Autodesk Inventor part; units mm, degrees
ref_plane "YZ Plane" through (0, 0, 0) normal (1, 0, 0) x (0, 1, 0)
ref_plane "XZ Plane" through (0, 0, 0) normal (0, 1, 0) x (-1, 0, 0)
ref_plane "XY Plane" through (0, 0, 0) normal (0, 0, 1) x (1, 0, 0)
sketch "草图1" plane through (0, 0, 0) normal (0, 0, 1) x (1, 0, 0)
  line L0 (-144.4444, 0) -> (-144.4444, 58)
  line L1 (-144.4444, 58) -> (-122.4444, 58)
  line L2 (-122.4444, 58) -> (-122.4444, 32)
  line L3 (-122.4444, 32) -> (-41.9444, 32)
  line L4 (-41.9444, 32) -> (-41.9444, 65)
  line L5 (-41.9444, 65) -> (-4.9444, 65)
  line L6 (-4.9444, 65) -> (-4.9444, 38)
  line L7 (-4.9444, 38) -> (30.0556, 38)
  line L8 (30.0556, 38) -> (30.0556, 0)
  line L9 (0, 0) -> (-166.6667, 0) construction
  line L10 (-144.4444, 0) -> (-144.4444, -58)
  line L11 (-144.4444, -58) -> (-122.4444, -58)
  line L12 (-122.4444, -58) -> (-122.4444, -32)
  line L13 (-122.4444, -32) -> (-41.9444, -32)
  line L14 (-41.9444, -32) -> (-41.9444, -65)
  line L15 (-41.9444, -65) -> (-4.9444, -65)
  line L16 (-4.9444, -65) -> (-4.9444, -38)
  line L17 (-4.9444, -38) -> (30.0556, -38)
  line L18 (30.0556, -38) -> (30.0556, 0)
  circle A0 centre (-106.5528, 0) radius 7.5
  circle A1 centre (-64.5976, 0) radius 7.5
  point P0 (-141.4444, -54)
  point P1 (-127.4444, -54)
  point P2 (-27.9137, -54)
  point P3 (-14.1378, -54)
  point P4 (-112.1204, -28)
  point P5 (-64.5976, -28)
  point P6 (-89.6514, -28)
  point P7 (-127.4444, -38)
  point P8 (-141.4444, -38)
  point P9 (-27.9137, -38)
  point P10 (-14.3619, -38)
  point P11 (-141.4444, 54)
  point P12 (-127.4444, 54)
  point P13 (-127.4444, 38)
  point P14 (-141.4444, 38)
  point P15 (-27.9137, 54)
  point P16 (-27.9137, 38)
  point P17 (-14.1378, 54)
  point P18 (-14.3619, 38)
  point P19 (-64.5976, 28)
  point P20 (-89.6514, 28)
  point P21 (-112.1204, 28)
  point P22 (-133.4444, 58)
  point P23 (-23.4444, 65)
  dimension "d0" = 22
  dimension "d1" = 37
  dimension "d3" = 32
  dimension "d4" = 38
  dimension "d5" = 35
  dimension "d6" = 58
  dimension "d7" = 15
  dimension "d8" = 15
  dimension "d29" = 28
  dimension "d30" = 28
  dimension "d31" = 28
  dimension "d36" = 110
  dimension "d96" = 33
extrude "拉伸1" add sketch "草图1" along normal blind 5
sketch "草图2" plane through (0, 0, 5) normal (0, 0, 1) x (1, 0, 0)
  circle A0 centre (-64.5976, 0) radius 7.5 construction
  circle A1 centre (-106.5528, 0) radius 7.5 construction
  line L0 (-144.4444, -58) -> (-144.4444, 58) construction
  line L1 (-144.4444, 58) -> (-122.4444, 58) construction
  line L2 (-122.4444, 58) -> (-122.4444, 32) construction
  line L3 (-122.4444, 32) -> (-41.9444, 32) construction
  line L4 (-41.9444, 32) -> (-41.9444, 65) construction
  line L5 (-41.9444, 65) -> (-4.9444, 65) construction
  line L6 (-4.9444, 65) -> (-4.9444, 38) construction
  line L7 (-4.9444, 38) -> (30.0556, 38) construction
  line L8 (30.0556, 38) -> (30.0556, -38) construction
  line L9 (30.0556, -38) -> (-4.9444, -38) construction
  line L10 (-4.9444, -38) -> (-4.9444, -65) construction
  line L11 (-4.9444, -65) -> (-41.9444, -65) construction
  line L12 (-41.9444, -65) -> (-41.9444, -32) construction
  line L13 (-41.9444, -32) -> (-122.4444, -32) construction
  line L14 (-122.4444, -32) -> (-122.4444, -58) construction
  line L15 (-122.4444, -58) -> (-144.4444, -58) construction
  line L16 (-164.7255, 0) -> (-80.9793, 0) construction
  point P0 (0, 0)
  point P1 (-141.4444, 55)
  point P2 (-125.4444, 55)
  point P3 (-38.4444, 61.5)
  point P4 (-8.4444, 61.5)
  point P5 (-38.4444, 37.5)
  point P6 (-8.4444, 37.5)
  point P7 (-125.4444, 41)
  point P8 (-141.4444, 41)
  point P9 (-141.4444, -55)
  point P10 (-125.4444, -55)
  point P11 (-38.4444, -61.5)
  point P12 (-8.4444, -61.5)
  point P13 (-38.4444, -37.5)
  point P14 (-8.4444, -37.5)
  point P15 (-125.4444, -41)
  point P16 (-141.4444, -41)
  dimension "d32" = 3
  dimension "d33" = 3
  dimension "d34" = 16
  dimension "d37" = 3
  dimension "d38" = 14
  dimension "d39" = 3
  dimension "d40" = 14
  dimension "d42" = 30
  dimension "d43" = 30
  dimension "d44" = 24
  dimension "d45" = 3.5
  dimension "d46" = 3.5
  dimension "d47" = 3.5
  dimension "d95" = 16
hole "孔2" at (-141.4444, 55, 5) at (-125.4444, 55, 5) at (-125.4444, 41, 5) at (-141.4444, 41, 5) at (-141.4444, -41, 5) at (-125.4444, -41, 5) at (-125.4444, -55, 5) at (-141.4444, -55, 5) direction (0, 0, -1) diameter 3.6 end through all
sketch "草图3" plane through (0, 0, 5) normal (0, 0, 1) x (1, 0, 0)
  circle A0 centre (-125.4444, -55) radius 1.8 construction
  circle A1 centre (-141.4444, -55) radius 1.8 construction
  circle A2 centre (-125.4444, 41) radius 1.8 construction
  circle A3 centre (-141.4444, 55) radius 1.8 construction
  circle A4 centre (-125.4444, 55) radius 1.8 construction
  circle A5 centre (-141.4444, 41) radius 1.8 construction
  circle A6 centre (-141.4444, -41) radius 1.8 construction
  circle A7 centre (-125.4444, -41) radius 1.8 construction
  circle A8 centre (-64.5976, 0) radius 7.5 construction
  circle A9 centre (-106.5528, 0) radius 7.5 construction
  line L0 (-144.4444, 58) -> (-144.4444, -58) construction
  line L1 (-144.4444, -58) -> (-122.4444, -58) construction
  line L2 (-122.4444, -58) -> (-122.4444, -32) construction
  line L3 (-122.4444, -32) -> (-41.9444, -32) construction
  line L4 (-41.9444, -32) -> (-41.9444, -65) construction
  line L5 (-41.9444, -65) -> (-4.9444, -65) construction
  line L6 (-4.9444, -65) -> (-4.9444, -38) construction
  line L7 (-4.9444, -38) -> (30.0556, -38) construction
  line L8 (30.0556, -38) -> (30.0556, 38) construction
  line L9 (30.0556, 38) -> (-4.9444, 38) construction
  line L10 (-4.9444, 38) -> (-4.9444, 65) construction
  line L11 (-4.9444, 65) -> (-41.9444, 65) construction
  line L12 (-41.9444, 65) -> (-41.9444, 32) construction
  line L13 (-41.9444, 32) -> (-122.4444, 32) construction
  line L14 (-122.4444, 32) -> (-122.4444, 58) construction
  line L15 (-122.4444, 58) -> (-144.4444, 58) construction
  line L16 (0, 0) -> (-184.5407, 0) construction
  point P0 (-139.9444, 25.8646)
  point P1 (-139.9444, 10.9473)
  point P2 (-108.7515, 25.8646)
  point P3 (-89.9847, 25.8646)
  point P4 (-70.7366, 25.8646)
  point P5 (-139.9444, -25.8646)
  point P6 (-139.9444, -10.9473)
  point P7 (-108.7515, -25.8646)
  point P8 (-89.9847, -25.8646)
  point P9 (-70.7366, -25.8646)
  point P10 (-139.9444, 0)
hole "孔3" at (-139.9444, 25.8646, 5) at (-139.9444, -25.8646, 5) at (-139.9444, 0, 5) direction (0, 0, -1) diameter 3.2 end through all
sketch "草图4" plane through (0, 0, 5) normal (0, 0, 1) x (1, 0, 0)
  circle A0 centre (-13.8026, 0) radius 7.5
  line L0 (0, 0) -> (-54.2498, 0) construction
  line L1 (-144.4444, 58) -> (-144.4444, -58) construction
  line L2 (30.0556, -38) -> (30.0556, 38) construction
  point P0 (-19.9444, 18.5)
  point P1 (17.0556, 18.5)
  point P2 (9.0556, 35)
  point P3 (-19.9444, -18.5)
  point P4 (17.0556, -18.5)
  point P5 (9.0556, -35)
  point P6 (-65.2677, 13.1999)
  point P7 (-65.2677, -14.7401)
  dimension "d62" = 15
  dimension "d67" = 37
  dimension "d68" = 50
  dimension "d69" = 18.5
  dimension "d70" = 35
  dimension "d71" = 21
  dimension "d94" = 27.94
extrude "拉伸2" cut sketch "草图4" against normal through all
sketch "草图5" plane through (0, 0, 5) normal (0, 0, 1) x (1, 0, 0)
  line L0 (30.0556, -38) -> (30.0556, 38)
  line L1 (0, 0) -> (-47.6944, 0) construction
  point P0 (26.0556, 29)
  point P1 (-43.9444, 29)
  point P2 (-43.7151, 20)
  point P3 (26.0556, -29)
  point P4 (-43.9444, -29)
  point P5 (-43.7151, -20)
  dimension "d81" = 70
  dimension "d83" = 4
  dimension "d84" = 29
  dimension "d85" = 20
  dimension "d86" = 29
hole "孔5" at (-43.9444, 29, 5) at (-43.9444, -29, 5) at (26.0556, 29, 5) at (26.0556, -29, 5) direction (0, 0, -1) diameter 3.2 end through all
hole "孔6" at (-38.4444, 61.5, 5) at (-8.4444, 61.5, 5) at (-38.4444, 37.5, 5) at (-8.4444, 37.5, 5) at (-38.4444, -37.5, 5) at (-8.4444, -37.5, 5) at (-8.4444, -61.5, 5) at (-38.4444, -61.5, 5) direction (0, 0, -1) diameter 4.2 end through all
sketch "草图6" plane through (0, 0, 5) normal (0, 0, 1) x (1, 0, 0)
  line L0 (-144.4444, 58) -> (-144.4444, -58)
  line L1 (0, 0) -> (-40.7503, 0) construction
  point P0 (-129.4444, 18.5)
  point P1 (-92.4444, 18.5)
  point P2 (-129.4444, -18.5)
  point P3 (-92.4444, -18.5)
  dimension "d104" = 15
  dimension "d105" = 37
  dimension "d106" = 18.5
  dimension "d107" = 18.5
hole "孔7" at (-129.4444, 18.5, 5) at (-92.4444, 18.5, 5) at (-129.4444, -18.5, 5) at (-92.4444, -18.5, 5) direction (0, 0, -1) diameter 3.2 end through all
sketch "草图7" plane through (0, 0, 5) normal (0, 0, 1) x (1, 0, 0)
  point P0 (0, 0)
  point P1 (11.1767, 22.7515)
  point P2 (17.9767, -25.8485)
  point P3 (-62.1233, 22.7515)
  point P4 (-64.6233, -25.2485)
  dimension "d115" = 48.6
  dimension "d116" = 6.8
  dimension "d117" = 73.3
  dimension "d118" = 48
  dimension "d119" = 2.5
hole "孔8" at (-64.6233, -25.2485, 5) at (17.9767, -25.8485, 5) direction (0, 0, -1) diameter 3.2 end through all
sketch "草图8" plane through (0, 0, 5) normal (0, 0, 1) x (1, 0, 0)
  line L0 (30.0556, 38) -> (-4.9444, 38)
  line L1 (0, 0) -> (93.7016, 0) construction
  line L2 (30.0556, -38) -> (30.0556, 38)
  line L3 (-41.9444, 32) -> (-122.4444, 32)
  point P0 (5.0556, 29)
  point P1 (-9.9444, 29)
  point P2 (5.0556, -29)
  point P3 (-9.9444, -29)
  point P4 (-111.5097, 25)
  point P5 (-111.5097, -25)
  dimension "d127" = 15
  dimension "d128" = 9
  dimension "d129" = 9
  dimension "d137" = 25
  dimension "d138" = 7
hole "孔9" at (5.0556, 29, 5) at (-9.9444, 29, 5) at (-9.9444, -29, 5) at (5.0556, -29, 5) at (-111.5097, 25, 5) at (-111.5097, -25, 5) direction (0, 0, -1) diameter 3.2 end through all
properties part number "底盘4.0" material "尼龙 6/6"
Could you check a few things on this model? Use its own coordinates, in mm. A direction names the side the tool comes from. Give positions to 0.01 mm unless a question says otherwise; leave off trailing zeros. Loops run counter-clockwise (first coordinate to the right, second up) from the corner with the lowest first, then second, coordinate; pieces in that order, holes last. Notation, with made-up numbers: (-7.75, 37.5) -> (9.25, 37.5) arc R18 cw to (9.25, 43.5) -> close; hole circle Ø6 at (-4.75, 41). An arc over 180 degrees is marked (long way). Return JSON: item names as keys, results as strings.
Item 1: If we section it at C-C on z = 2.45: Count the separate pieces of the cut face and the enclosed holes in it, plus the area to 3 significant figures.
Geometry results:
{"separate pieces": "1", "enclosed holes": "38", "area": "14,300 mm²"}
Item 2: Which directions (+Z, -Z, +X, -X, +Y, -Y) give clear straight access to the entire face, cutting with the end or side of a thin tool? Please do faces 1 (the flat face through (-41.944, -48, 2)), 2 (the cylindrical face through (-139.687, 55.39, 2.465)), 3 (the flat face through (-134, 58, 2)).
Geometry results:
{"face 1": "+Z, -Z, -Y", "face 2": "+Z, -Z", "face 3": "+Z, -Z, -X, +Y"}
Item 3: I'm going to push flat-ended pins straight in: pin 1 (2.5 mm diameter, centred on x = -91.5, z = 2, fed in from -Y); pin 2 (1.9 mm diameter, centred on x = 26.06, y = -29, fed in from +Z); pin 3 (1.5 mm diameter, centred on x = 9.5, z = 1.5, fed in from +Y). Where does each tip first touch, or does it pass through?
Geometry results:
{"pin 1": "stops at y = -32", "pin 2": "passes through", "pin 3": "stops at y = 38"}
Item 4: I need wall thicknesses on L1, parallel to X at y = 55, z = 2.75; L2, parallel to X at y = 37.5, z = 4.2; L3, parallel to Y at x = -38.5, z = 2.1. Which ranges of each line are inside material? Lowest first, please. Write a range as from..to.
Geometry results:
{"L1": "x = -144.44..-143.24, -139.64..-127.24, -123.64..-122.44, -41.94..-4.94", "L2": "x = -144.44..-122.44, -41.94..-40.54, -36.34..-10.54, -6.34..30.06", "L3": "y = -65..-63.6, -59.4..-39.6, -35.4..35.4, 39.6..59.4, 63.6..65"}
Item 5: If we section it at A-A on y = -61.5: List the corners of the cut face in (x, z) for me.
Geometry results:
{"outline": "(-41.94, 0) -> (-40.54, 0) -> (-40.54, 5) -> (-41.94, 5) -> close; (-36.34, 0) -> (-10.54, 0) -> (-10.54, 5) -> (-36.34, 5) -> close; (-6.34, 0) -> (-4.94, 0) -> (-4.94, 5) -> (-6.34, 5) -> close"}
Item 6: We'd pull the mould along X, two halves only. Please class faces 4 (the cylindrical face through (-38.5, -35.4, 2.5)), 5 (the flat face through (12, -38, 2)), 6 (the flat face through (-4.944, 52, 2)): +X half, -X half, draft (parallel to the pull), parting line (faces both ways), or undercut.
Geometry results:
{"face 4": "undercut", "face 5": "draft", "face 6": "+X half"}
Item 7: If we section it at B-B on x = -14: List the corners of the cut face in (y, z) for me.
Geometry results:
{"outline": "(-65, 0) -> (-7.5, 0) -> (-7.5, 5) -> (-65, 5) -> close; (7.5, 0) -> (65, 0) -> (65, 5) -> (7.5, 5) -> close"}
